The figure shows three views and two pictorial views of one solid part (mm, origin at its lowest corner). Answer the questions. A direction names the side the tool comes from. Give positions to 0.01 mm unless a question says otherwise; leave off trailing zeros. Loops run counter-clockwise (first coordinate to the right, second up) from the corner with the lowest first, then second, coordinate; pieces in that order, holes last. Notation, with made-up numbers: (62.25, 57) - (80.25, 57) arc R32 ccw to (80.25, 93) - close; hole circle Ø8 at (-23.5, 52). An arc over 180 degrees is marked (long way). Write item = value, one per line.
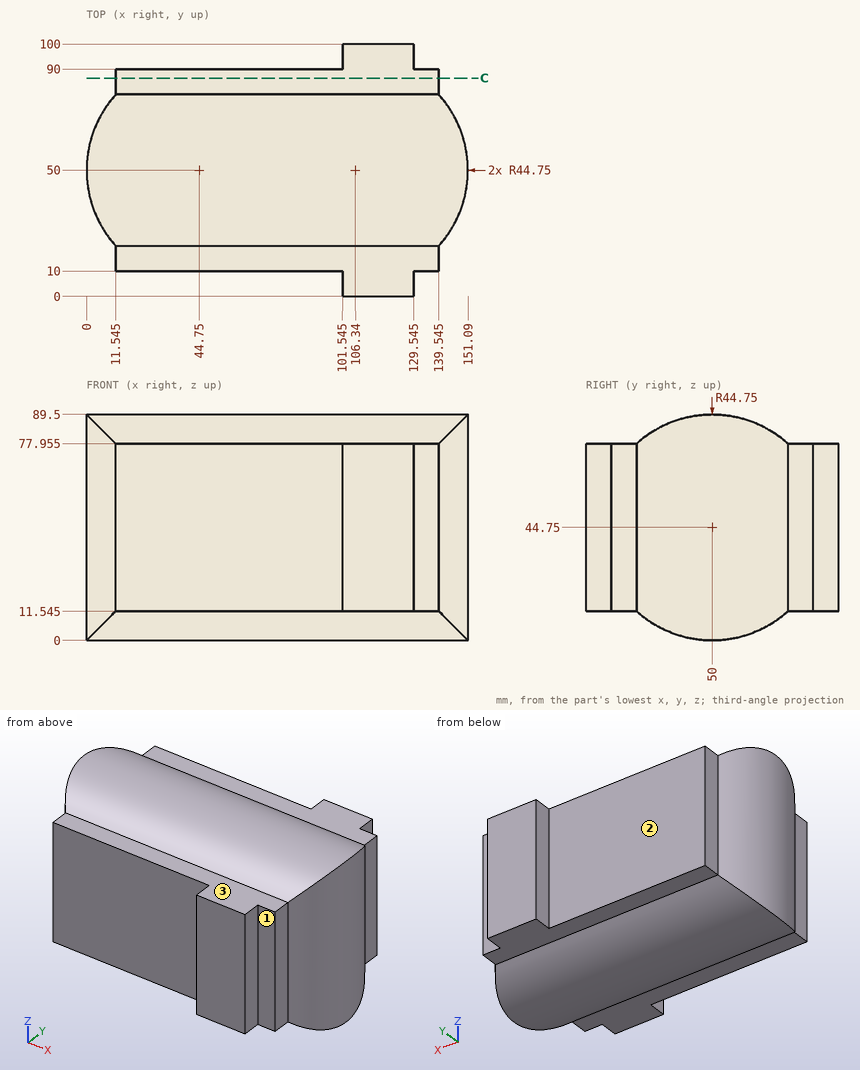
1) Each of these flat-tipped pins is pushed along its axis until it touches: P1, Ø4, axis at y = 83.5, z = 10.5, coming from the +X side (3 decimals); P2, Ø6, axis at y = 30, z = 20, coming from the +X side (1 decimal); P3, Ø2, axis at x = 87, z = 79, coming from the +Y side. Where does it stop, or does it pass through?
Output:
P1 = 139.545
P2 = 147.7
P3 = 79.95
2) A tool of negligible diameter and unlimited length cuts with its end or side. For the marked faces 1, 2 and 3, from which of +Z, -Z, +X, -X, +Y, -Y can it reach the whole face along a straight path? Write none if from no direction.
Output:
face_1 = +Z, -Z, +X, -Y
face_2 = +Z, -Z, -X, +Y
face_3 = +Z, +X, -X, -Y
3) A cutting plane is placed at C-C on y = 86.5. Determine the outline of the cut face in (x, z) (1 decimal).
Output:
outline = (11.5, 11.5) - (139.5, 11.5) - (139.5, 78) - (11.5, 78) - close
4) Find the intervals of material crossed by probe 1 along Y at (x, z) = (44, 56); probe 2 along Z at (x, y) = (30, 84) (1 decimal); probe 3 along X at (y, z) = (13, 59.5) (1 decimal), in increasing order.
Output:
probe_1 = 10 to 90
probe_2 = 11.5 to 78
probe_3 = 11.5 to 139.5
